from build123d import *

# Parameters (mm, degrees)
F1_DEPTH = 30
F2_R     = 1
F3_DEPTH = 15


with BuildPart() as f1:
    # F0 (on Top) → F1 (new body)
    with BuildSketch(Plane.XY):
        with BuildLine():
            Line((0, 45), (0, 0))
            Line((0, 0), (4.900002, 0))
            Line((4.900002, 0), (4.900002, 40))
            Line((4.900002, 40), (29.900002, 40))
            Line((29.900002, 40), (29.900002, 26))
            Line((29.900002, 26), (27.900002, 26))
            Line((27.900002, 26), (27.900002, 21))
            Line((27.900002, 21), (30, 21))
            ThreePointArc((30, 21), (33.535534, 22.464466), (35, 26))
            Line((35, 26), (35, 43))
            ThreePointArc((35, 43), (34.414214, 44.414214), (33, 45))
            Line((33, 45), (4.900002, 45))
            Line((4.900002, 45), (4.900002, 50))
            Line((4.900002, 50), (30, 50))
            Line((30, 50), (30, 55))
            Line((30, 55), (0, 55))
            Line((0, 55), (0, 45))
        make_face()
    extrude(amount=F1_DEPTH)

    # F2 (on face) → F3 (cut)
    with BuildSketch(Plane.YZ.offset(30)):
        with Locations((52.5, 15)):
            Circle(F2_R)
    extrude(amount=-F3_DEPTH, mode=Mode.SUBTRACT)


solid = f1.part
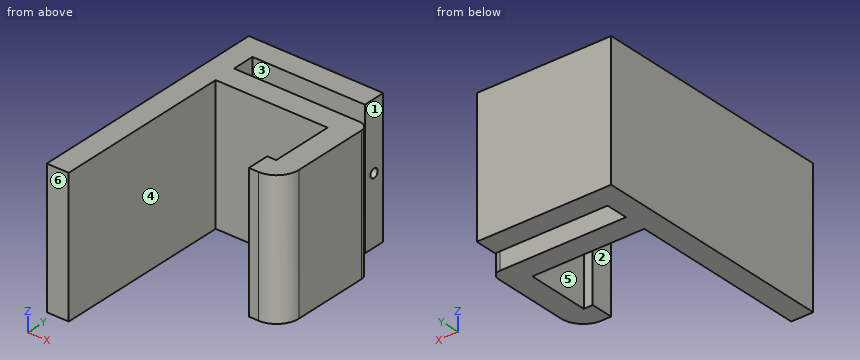
Work out the finished part from the listing and answer in its coordinate system (mm). Face numbers are marked on the shaded views. A direction names the side the tool comes from. Coordinates: 2 decimals unless noted, no trailing zeros. Write each loop counter-clockwise with the first axis right and the second up, starting at its lowest first coordinate (ties: lowest second). Pieces come first, ordered by that corner, then holes. Notation, with made-up numbers: M 7.25,75.5 L 25.25,75.5 A17 cw 25.25,82.5 Z; hole C 27.5,10 d7. An arc over 180 degrees is marked long. Write item = value, one per line.
1. The part is cut by section A-A (x = 25). Determine the outline of the cut face in (y, z), then the cut area to 3 significant figures.
Solution:
outline = M 40,0 L 45,0 L 45,30 L 40,30 Z; M 50,0 L 55,0 L 55,30 L 50,30 Z; hole C 52.5,15 d2
area = 297 mm2
2. The part is cut by section B-B (y = 23). Determine the outline of the cut face in (x, z), then the cut area to 3 significant figures.
Solution:
outline = M 0,0 L 4.9,0 L 4.9,30 L 0,30 Z; M 27.9,0 L 34,0 L 34,30 L 27.9,30 Z
area = 330 mm2
3. Flat-ended cylindrical pins translate along their axes: pin 1 (1.5 mm diameter, centred on y = 46.5, z = 16, fed in from +X); pin 2 (1.5 mm diameter, centred on y = 51.5, z = 11, fed in from +X); pin 3 (12.5 mm diameter, centred on x = 21, z = 9.5, fed in from -Y). Find the tip coordinate at first contact, or state that the pin passes through.
Solution:
pin_1 = 4.9
pin_2 = 30
pin_3 = 40
4. The part is cut by section C-C (z = 6.5). Determine the outline of the cut face in (x, y).
Solution:
outline = M 0,0 L 4.9,0 L 4.9,40 L 29.9,40 L 29.9,26 L 27.9,26 L 27.9,21 L 30,21 A5 ccw 35,26 L 35,43 A2 ccw 33,45 L 4.9,45 L 4.9,50 L 30,50 L 30,55 L 0,55 Z
5. Straight lines are drawn through the part: line 1 (Y direction, x = 10.5, z = 22.5); line 2 (Z direction, x = 23.25, y = 52.5); line 3 (X direction, y = 29.5, z = 16.5). For each, find the intervals that lie inside material, in ascending order. Write a range as from..to.
Solution:
line_1 = 40..45, 50..55
line_2 = 0..14, 16..30
line_3 = 0..4.9, 29.9..35
6. For the marked faces 1, 2 and 3, determine the directions among +Z, -Z, +X, -X, +Y, -Y from which every point of the face is accessible in a straight line to the end or side of a thin tool.
Solution:
face_1 = +Z, -Z, +X, +Y
face_2 = +Z, -Z, -Y
face_3 = +Z, -Z, +X
7. The part is cut by section D-D (x = 9.5). Determine the outline of the cut face in (y, z), then the cut area to 3 significant figures.
Solution:
outline = M 40,0 L 45,0 L 45,30 L 40,30 Z; M 50,0 L 55,0 L 55,30 L 50,30 Z
area = 300 mm2
8. Determine the mould class of the marked faces 4, 5 and 6 for opening direction Y: released by +Y, released by -Y, zero draft, split by the parting line, or undercut.
Solution:
face_4 = zero draft
face_5 = undercut
face_6 = released by -Y
